Autodesk Inventor part; units mm, degrees
ref_plane "YZ Plane" through (0, 0, 0) normal (1, 0, 0) x (0, 1, 0)
ref_plane "XZ Plane" through (0, 0, 0) normal (0, 1, 0) x (-1, 0, 0)
ref_plane "XY Plane" through (0, 0, 0) normal (0, 0, 1) x (1, 0, 0)
sketch "Sketch1" plane through (0, 0, 0) normal (0, 1, 0) x (-1, 0, 0)
  line L0 (139.7, 1219.2) -> (-139.7, 1219.2)
  line L1 (-139.7, 1219.2) -> (-139.7, -1219.2)
  line L2 (-139.7, -1219.2) -> (139.7, -1219.2)
  line L3 (139.7, -1219.2) -> (139.7, 1219.2)
  line L4 (139.7, 1219.2) -> (-139.7, -1219.2) construction
  line L5 (-139.7, 1219.2) -> (139.7, -1219.2) construction
  point P0 (0, 0)
  dimension "d0" = 279.4
  dimension "d1" = 2438.4
extrude "Extrusion1" add sketch "Sketch1" along normal blind 139.7
sketch "Sketch3" plane through (-139.7, 0, -1219.2) normal (-1, 0, 0) x (0, 0, 1)
  line L0 (2438.4, 139.7) -> (0, 139.7) construction
  line L1 (1219.2, 139.7) -> (1219.2, 0) construction
  line L2 (1219.2, 0) -> (1219.2, 25.4) construction
  line L3 (1219.2, 25.4) -> (0, 25.4)
  line L4 (1219.2, 25.4) -> (2438.4, 25.4)
  line L5 (2438.4, 0) -> (0, 0) construction
  ellipse E0 centre (1219.2024, 69.8468) end of major axis (1342.5189, 69.8468) minor radius 69.85 (1317.8532, 111.7586) -> (1120.5517, 111.7586) ccw
  line L6 (1219.2024, 69.8468) -> (1219.2024, 176.8167) construction
  line L7 (0, 69.85) -> (0, 127.0895)
  line L8 (2438.4, 127.0895) -> (2438.4, 57.2395)
  arc A0 (750.1497, 98.2079) -> (717.7137, 104.389) centre (727.3807, 66.9219) ccw
  arc A1 (0, 69.85) -> (208.3969, 123.3364) centre (0, 502.5771) ccw
  arc A2 (276.8498, 123.3364) -> (208.3969, 123.3364) centre (242.6233, 69.85) ccw
  arc A3 (487.68, 69.85) -> (717.7137, 104.389) centre (471.9739, 957.7485) ccw
  line L9 (135.5865, 91.6403) -> (352.0961, 91.6403) construction
  arc A4 (276.8498, 123.3364) -> (487.68, 69.85) centre (491.8688, 528.6244) ccw
  line L10 (1763.8663, 33.8803) -> (1763.8663, 113.409) construction
  ellipse E1 centre (1763.8663, 33.8803) end of major axis (1865.4663, 33.8803) minor radius 57.271 (1850.0792, 64.183) -> (1693.5763, 75.2333) ccw
  arc A5 (1520.0263, 33.8803) -> (1693.5763, 75.2333) centre (1529.4777, 379.0674) ccw
  arc A6 (975.36, 25.4) -> (1120.5517, 111.7586) centre (657.8319, 724.4807) ccw
  arc A7 (750.1497, 98.2079) -> (975.36, 25.4) centre (973.9324, 405.6999) ccw
  arc A8 (1317.8532, 111.7586) -> (1520.0263, 33.8803) centre (1554.8027, 425.5214) ccw
  arc A9 (2236.968, 117.8247) -> (2124.6268, 99.2248) centre (2194.56, 25.4) ccw
  arc A10 (1850.0792, 64.183) -> (1950.8132, 25.4) centre (1950.8132, 175.6133) ccw
  arc A11 (1950.8132, 25.4) -> (2124.6268, 99.2248) centre (1938.6597, 295.5405) ccw
  line L11 (2236.968, 117.8247) -> (2438.4, 25.4)
  line L12 (2438.4, 57.2395) -> (2438.4, 25.4)
  line L13 (1219.2, 127.0895) -> (1219.2024, 127.0895)
  line L14 (1219.2, 127.0895) -> (1219.2024, 127.0895)
  line L15 (1219.2, 127.0895) -> (1219.2024, 127.0895)
  line L16 (2438.4, 0) -> (2438.4, 139.7)
  line L17 (2438.4, 127.0895) -> (2438.4, 139.7)
  line L18 (2438.4, 139.7) -> (0, 139.7)
  line L19 (0, 0) -> (0, 139.7)
  line L20 (0, 127.0895) -> (0, 139.7)
  point P0 (729.1332, 155.8475)
  point P1 (243.84, 164.183)
  point P2 (1494.3481, 127.0895)
  dimension "d24" = 101.6
  dimension "d16" = 25.4
  dimension "d23" = 216.5096
extrude "Extrusion2" cut sketch "Sketch3" against normal through all contours A7 A0 A3 A4 A2 A1 L7 L19 L18 L16 L8 L12 L11 A9 A11 A10 E1 A5 A8 E0 A6
properties part number "landscape for mars rover"
Read the model definition and answer for the solid it produces. Units are mm, in the model's axes. A direction names the side the tool comes from. Give positions to 0.01 mm unless a question says otherwise; leave off trailing zeros. Loops run counter-clockwise (first coordinate to the right, second up) from the corner with the lowest first, then second, coordinate; pieces in that order, holes last.
Item 1: Each of these flat-tipped pins is pushed along its axis until it touches: pin 1 Ø5 at (x, z) = (-90, 162.5) entering from +Y; pin 2 Ø1.5 at (x, z) = (-88, 570.5) entering from +Y; pin 3 Ø12 at (x, z) = (39.5, -424.5) entering from +Y. Where does it stop, or does it pass through?
Item 2: The mould has two halves that part along Z. Classify faces 3 (the cylindrical face through (-1.956, 79.314, -616.982)), 4 (the cylindrical face through (-1.96, 83.06, -1113.1)), 5 (the flat face through (-1.96, 72.26, 1117.07)): released by +Z, released by -Z, zero draft, split by the parting line, or undercut.
Item 3: The part is cut by section B-B (z = -771). Write down the section's boundary in (x, y).
Item 4: Find the intervals of material crossed by line 1 along Z through (x, y) = (-88.5, 112.5); line 2 along Z through (x, y) = (-4, 113); line 3 along X through (y, z) = (66, -460), in increasing order.
Item 5: For faces 1 (the flat face through (2, 0, 17)), 2 (the cylindrical face through (-1.96, 84.3, -841.64)), determine the directions among +Z, -Z, +X, -X, +Y, -Y from which every point of the face is accessible in a straight line to the end or side of a thin tool.
Item 6: The part is cut by section A-A (z = 123). Write down the section's boundary in (x, y), and give its area (3 significant figures).
Taken from the geometry:
1. pin 1: stops at y = 73.73
1. pin 2: stops at y = 89.38
1. pin 3: stops at y = 73.56
2. face 3: undercut
2. face 4: released by -Z
2. face 5: released by +Z
3. outline: (-139.7, 0) - (139.7, 0) - (139.7, 71.91) - (-139.7, 71.91) - close
4. line 1: z = -1031.87 to -920.55, -97.65 to 97.66, 922.88 to 1029.37
4. line 2: z = -1030.83 to -921.62, -96.97 to 96.97, 923.72 to 1028.28
4. line 3: x = -139.7 to 139.7
5. face 1: +Z, -Z, +X, -X, -Y
5. face 2: +X, -X, +Y
6. outline: (-139.7, 0) - (139.7, 0) - (139.7, 94.78) - (-139.7, 94.78) - close
6. area: 26,500 mm2
